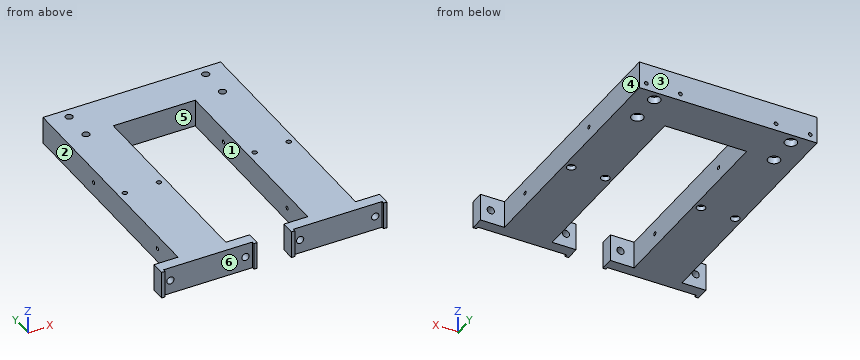
```python
from build123d import *

# Parameters (mm, degrees)
SKETCH1_W                                        = 165.1
SKETCH1_H                                        = 241.3
BOSS_EXTRUDE1_DEPTH                              = 25.4
SKETCH2_W                                        = 76.2
SKETCH2_H                                        = 203.2
CUT_EXTRUDE1_DEPTH                               = 149.378182358
SKETCH7_W                                        = 88.9
SKETCH7_H                                        = 12.7
BOSS_EXTRUDE4_DEPTH                              = 25.4
SKETCH8_W                                        = 82.55
SKETCH8_H                                        = 25.4
CUT_EXTRUDE4_DEPTH                               = 2.54
F_1_4_CLEARANCE_HOLE1_D                          = 6.7564
F_1_4_CLEARANCE_HOLE1_DEPTH                      = 10.16
CBORE_FOR_1_4_SOCKET_HEAD_CAP_SCREW1_D           = 6.7564
CBORE_FOR_1_4_SOCKET_HEAD_CAP_SCREW1_CBORE_D     = 11.1125
CBORE_FOR_1_4_SOCKET_HEAD_CAP_SCREW1_CBORE_DEPTH = 6.35
F_8_32_TAPPED_HOLE1_D                            = 3.4544
F_8_32_TAPPED_HOLE1_DEPTH                        = 12.7
F_8_32_TAPPED_HOLE1_TIP                          = 1.037806461
CBORE_FOR_8_SOCKET_HEAD_CAP_SCREW1_D             = 4.4958
CBORE_FOR_8_SOCKET_HEAD_CAP_SCREW1_CBORE_D       = 7.9375
CBORE_FOR_8_SOCKET_HEAD_CAP_SCREW1_CBORE_DEPTH   = 4.1656
F_8_32_TAPPED_HOLE2_D                            = 3.4544
F_8_32_TAPPED_HOLE2_DEPTH                        = 44.45


with BuildPart() as part:
    # Sketch1 → Boss-Extrude1 (new body)
    with BuildSketch(Plane.XY):
        Rectangle(SKETCH1_W, SKETCH1_H)
    extrude(amount=BOSS_EXTRUDE1_DEPTH)

    # Sketch2 → Cut-Extrude1 (cut, through all)
    with BuildSketch(Plane.XY.offset(25.4)):
        with Locations((0, -19.05)):
            Rectangle(SKETCH2_W, SKETCH2_H)
    extrude(amount=-CUT_EXTRUDE1_DEPTH, mode=Mode.SUBTRACT)

    # Sketch7 → Boss-Extrude4 (add)
    with BuildSketch(Plane.XY.offset(25.4)):
        with Locations((-60.325, -114.3)):
            Rectangle(SKETCH7_W, SKETCH7_H)
    boss_extrude4 = extrude(amount=-BOSS_EXTRUDE4_DEPTH)

    # Sketch8 → Cut-Extrude4 (cut)
    with BuildSketch(Plane(origin=(0, -120.65, 0), x_dir=(-1, 0, 0), z_dir=(0, -1, 0))):
        with Locations((60.325, -12.7)):
            Rectangle(SKETCH8_W, SKETCH8_H)
    cut_extrude4 = extrude(amount=-CUT_EXTRUDE4_DEPTH, mode=Mode.SUBTRACT)

    # Mirror3: Boss-Extrude4, Cut-Extrude4 across plane
    add(boss_extrude4.mirror(Plane(origin=(0, 0, 0), x_dir=(0, 0, 1), z_dir=(1, 0, 0))))
    add(cut_extrude4.mirror(Plane(origin=(0, 0, 0), x_dir=(0, 0, 1), z_dir=(1, 0, 0))), mode=Mode.SUBTRACT)

    # 1/4 Clearance Hole1
    with Locations(Plane(origin=(0, -107.95, 0), x_dir=(1, 0, 0), z_dir=(0, 1, 0))):
        with Locations((-95.25, -12.7), (-25.4, -12.7), (25.4, -12.7), (95.25, -12.7)):
            Hole(F_1_4_CLEARANCE_HOLE1_D / 2, depth=F_1_4_CLEARANCE_HOLE1_DEPTH)

    # CBORE for 1/4 Socket Head Cap Screw1 (through all)
    with Locations(Plane(origin=(0, 0, 0), x_dir=(-1, 0, 0), z_dir=(0, 0, -1))):
        with Locations((-63.5, 111.125), (-63.5, 82.55), (63.5, 111.125), (63.5, 82.55)):
            CounterBoreHole(CBORE_FOR_1_4_SOCKET_HEAD_CAP_SCREW1_D / 2, CBORE_FOR_1_4_SOCKET_HEAD_CAP_SCREW1_CBORE_D / 2, CBORE_FOR_1_4_SOCKET_HEAD_CAP_SCREW1_CBORE_DEPTH)

    # #8-32 Tapped Hole1
    with Locations(Plane(origin=(0, 120.65, 0), x_dir=(1, 0, 0), z_dir=(0, 1, 0))):
        with Locations((-76.2, -6.35), (-44.45, -6.35), (44.45, -6.35), (76.2, -6.35)):
            Hole(F_8_32_TAPPED_HOLE1_D / 2, depth=F_8_32_TAPPED_HOLE1_DEPTH)
            with Locations((0, 0, -(F_8_32_TAPPED_HOLE1_DEPTH + F_8_32_TAPPED_HOLE1_TIP / 2))):  # 118° drill point
                Cone(0, F_8_32_TAPPED_HOLE1_D / 2, F_8_32_TAPPED_HOLE1_TIP, mode=Mode.SUBTRACT)

    # CBORE for #8 Socket Head Cap Screw1 (through all)
    with Locations(Plane(origin=(0, 0, 0), x_dir=(-1, 0, 0), z_dir=(0, 0, -1))):
        with Locations((-76.2, -6.35), (-44.45, -6.35), (44.45, -6.35), (76.2, -6.35)):
            CounterBoreHole(CBORE_FOR_8_SOCKET_HEAD_CAP_SCREW1_D / 2, CBORE_FOR_8_SOCKET_HEAD_CAP_SCREW1_CBORE_D / 2, CBORE_FOR_8_SOCKET_HEAD_CAP_SCREW1_CBORE_DEPTH)

    # #8-32 Tapped Hole2
    with Locations(Plane.ZY.offset(82.55)):
        with Locations((12.7, -73.025), (12.7, 34.925)):
            f_8_32_tapped_hole2 = Hole(F_8_32_TAPPED_HOLE2_D / 2, depth=F_8_32_TAPPED_HOLE2_DEPTH)

    # Mirror4: #8-32 Tapped Hole2 across plane
    add(f_8_32_tapped_hole2.mirror(Plane(origin=(0, 0, 0), x_dir=(0, 0, 1), z_dir=(1, 0, 0))), mode=Mode.SUBTRACT)


solid = part.part
```
For this review, take the finished solid that the model builds, in its own axes (mm). Face numbers are marked on the shaded views. A direction names the side the tool comes from. Coordinates: 2 decimals unless noted, no trailing zeros. Loops run counter-clockwise (first coordinate to the right, second up) from the corner with the lowest first, then second, coordinate; pieces in that order, holes last.
1. Add section A-A, the plane x = 95.25. Give the boundary of the cut face in (y, z), then the cut area to 3 significant figures.
2. For line 1 (X direction, y = -112.75, z = 12.7) (3 decimals); line 2 (Z direction, x = 76.2, y = 111.5); line 3 (X direction, y = -43, z = 14), list the stretches that pass through material, from the lowest coordinate up.
3. Insertion check: P1, Ø12, axis at x = 20.5, z = 6.5, coming from the -Y side; P2, Ø3.5, axis at x = 61, y = 82.5, coming from the -Z side; P3, Ø10, axis at y = 24, z = 16.5, coming from the -X side; P4, Ø1.5, axis at x = 46, z = 22.5, coming from the -Y side. Each pin has a flat end and moves straight along its axis. Give the tip position at first contact, or say it passes through.
4. For the marked faces 4, 5 and 6, list the 3-axis set-ups (+Z, -Z, +X, -X, +Y, -Y) from which the entire face can be reached by the end or side of a thin tool; tool diameter is ignored.
5. Add section D-D, the plane z = 21.75. Count the separate pieces of the cut face and the enclosed holes in it, then the cut area to 3 significant figures.
6. Mouldability with a two-part tool opening along Y and no side actions: class the marked faces 1, 2 and 3 as +Y half, -Y half, draft (parallel to the pull), parting line (faces both ways), or undercut.
7. Add section B-B, the plane x = 25.4. Give the boundary of the cut face in (y, z).
8. Add section C-C, the plane y = -87. Give the boundary of the cut face in (x, z), then the cut area to 3 significant figures.
Result:
1. outline: (-118.11, 0) - (-107.95, 0) - (-107.95, 9.32) - (-118.11, 9.32) - close; (-118.11, 16.08) - (-107.95, 16.08) - (-107.95, 25.4) - (-118.11, 25.4) - close
1. area: 189 mm2
2. line 1: x = -104.775 to -98.628, -91.872 to -28.778, -22.022 to -15.875, 15.875 to 22.022, 28.778 to 91.872, 98.628 to 104.775
2. line 2: z = 0 to 4.62, 8.08 to 25.4
2. line 3: x = -82.55 to -38.1, 38.1 to 82.55
3. P1: stops at y = -120.65
3. P2: stops at z = 6.35
3. P3: stops at x = -82.55
3. P4: stops at y = -118.11
4. face 4: +Z, -Z, +X, +Y
4. face 5: +Z, -Z
4. face 6: +Z, -Z, -Y
5. separate pieces: 1
5. enclosed holes: 8
5. area: 24,900 mm2
6. face 1: undercut
6. face 2: draft
6. face 3: +Y half
7. outline: (-118.11, 0) - (-107.95, 0) - (-107.95, 9.32) - (-118.11, 9.32) - close; (-118.11, 16.08) - (-107.95, 16.08) - (-107.95, 25.4) - (-118.11, 25.4) - close; (82.55, 0) - (120.65, 0) - (120.65, 25.4) - (82.55, 25.4) - close
8. outline: (-82.55, 0) - (-38.1, 0) - (-38.1, 25.4) - (-82.55, 25.4) - close; (38.1, 0) - (82.55, 0) - (82.55, 25.4) - (38.1, 25.4) - close
8. area: 2,260 mm2
